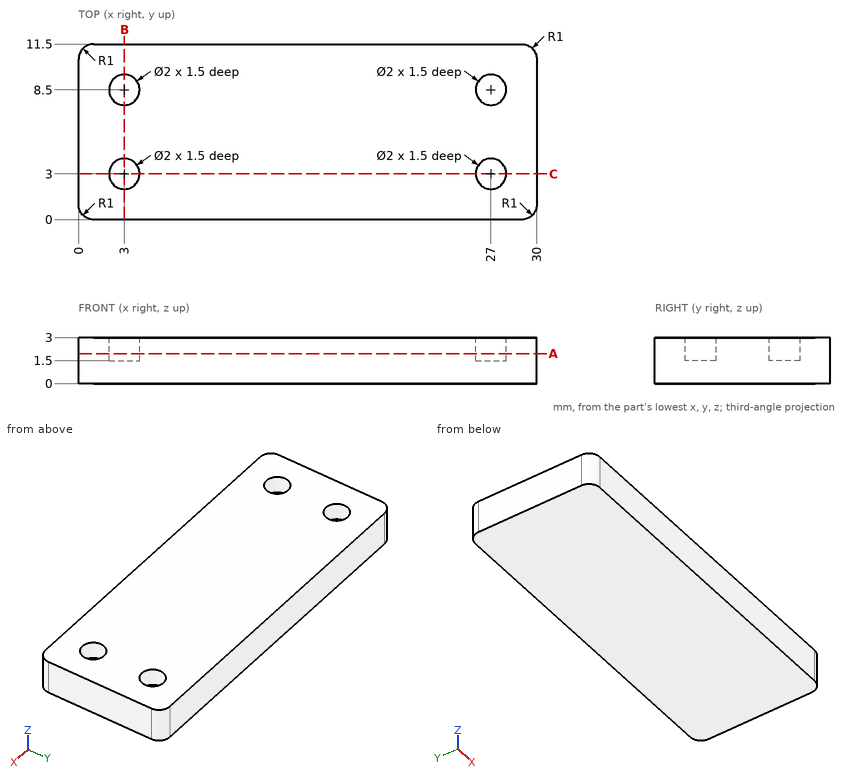
The drawing under review shows one solid part. Ordinate dimensions are in mm from its lowest x, y, z. Round coordinates to 2 decimals unless told otherwise and drop trailing zeros. Write each loop counter-clockwise with the first axis right and the second up, starting at its lowest first coordinate (ties: lowest second). Pieces come first, ordered by that corner, then holes. Notation, with made-up numbers: M 14.25,-32.5 L 18.25,-32.5 A33 ccw 18.25,5.5 Z; hole C -19.5,6 d11. An arc over 180 degrees is marked long. One line per item, written item: value. Start each with the question number.
(1) We need section B-B (x = 3). Give the boundary of the cut face in (y, z), and give its area (3 significant figures).
(2) Insertion check: pin 1 (1.6 mm diameter, centred on x = 26.5, y = 8, fed in from +Z); pin 2 (1 mm diameter, centred on x = 27, y = 3, fed in from +Z). Each pin has a flat end and moves straight along its axis. Give the tip position at first contact, or say it passes through.
(3) We need section A-A (z = 1.95). Give the boundary of the cut face in (x, y).
(4) Wall thickness on line 1 (X direction, y = 8.5, z = 2.55); line 2 (Y direction, x = 3, z = 2.1); line 3 (Y direction, x = 27.5, z = 2.8): over which ranges is each line inside the solid? List them lowest first.
(5) We need section C-C (y = 3). Give the boundary of the cut face in (x, z).
Result:
1. outline: M 0,0 L 11.5,0 L 11.5,3 L 9.5,3 L 9.5,1.5 L 7.5,1.5 L 7.5,3 L 4,3 L 4,1.5 L 2,1.5 L 2,3 L 0,3 Z
1. area: 28.5 mm²
2. pin 1: z = 3
2. pin 2: z = 1.5
3. outline: M 0,1 A1 ccw 1,0 L 29,0 A1 ccw 30,1 L 30,10.5 A1 ccw 29,11.5 L 1,11.5 A1 ccw 0,10.5 Z; hole C 3,3 d2; hole C 3,8.5 d2; hole C 27,3 d2; hole C 27,8.5 d2
4. line 1: 0 to 2, 4 to 26, 28 to 30
4. line 2: 0 to 2, 4 to 7.5, 9.5 to 11.5
4. line 3: 0 to 2.13, 3.87 to 7.63, 9.37 to 11.5
5. outline: M 0,0 L 30,0 L 30,3 L 28,3 L 28,1.5 L 26,1.5 L 26,3 L 4,3 L 4,1.5 L 2,1.5 L 2,3 L 0,3 Z
